The model under review builds one solid part; all positions refer to its coordinate system, in mm. A direction names the side the tool comes from. Round coordinates to 2 decimals unless told otherwise and drop trailing zeros. Order: outer loops, then holes, each group sorted by start corner. A loop starts at its lowest first (then second) coordinate and runs counter-clockwise, first axis right, second up.
1) Consider section D-D (y = 0). Give the number of separate pieces and of enclosed holes in the cut face, then the cut area to 3 significant figures.
2) Clearance check with flat-ended pins moving along their axes: P1, Ø1, axis at x = -20.5, y = 1, coming from the +Z side; P2, Ø1, axis at x = 3, y = -2, coming from the +Z side. State where each tip first meets the part, or that it passes through.
3) Consider section B-B (x = 9.5). Give the boundary of the cut face in (y, z).
4) Consider section C-C (z = 5.5). Give the boundary of the cut face in (x, y), then the cut area to 3 significant figures.
5) Consider section A-A (z = 18). Give the boundary of the cut face in (x, y).
6) To check wall thickness, follow L1, parallel to X at y = 0, z = 14.75; L2, parallel to Y at x = -18.5, z = 0.9; L3, parallel to Z at x = -21.5, y = 3.75. State the ranges of each line that lie inside material, in increasing order.
7) Machinability: for faces 4 (the face through (-5, 11, 12)), 5 (the face through (-16, 8.5, 8)), 6 (the face through (0, 0, 4)), 7 (the face through (10.63, -2.82, 15.67)), which of the approach directions +Z, -Z, +X, -X, +Y, -Y give a long, thin tool a straight path to every point of the face, cutting with its end or side? Answer none if there is none.
8) Mouldability with a two-part tool opening along X and no side actions: class faces 1 (the face through (20.4, 4.19, 9.98)), 2 (the face through (0, 0, 0)), 3 (the face through (32.5, 0, 10)) as pulls with the +X half, pulls with the -X half, needs draft (parallel to the pull), parting line crosses it, or undercut.
from build123d import *

# Parameters (mm, degrees)
SKETCH_W             = 65
SKETCH_H             = 24.999
PAD_DEPTH            = 19.999
POCKET_DEPTH         = 20.9992
POCKET001_DEPTH      = 20.9992
SKETCH003_R          = 10.9995
POCKET002_DEPTH      = 15.9992
SKETCH004_W          = 9.9995
SKETCH004_H          = 15.9992
POCKET003_DEPTH      = 12.5005
POCKET003_DEPTH_BACK = -12.5005
SKETCH005_R          = 3
POCKET004_DEPTH      = 20
CHAMFER_SIZE         = 1.5


with BuildPart() as part:
    # Sketch → Pad (new body)
    with BuildSketch(Plane.XY):
        Rectangle(SKETCH_W, SKETCH_H)
    extrude(amount=PAD_DEPTH)

    # Sketch001 → Pocket (cut)
    with BuildSketch(Plane.XZ.offset(-8.4997)):
        Polygon((0, 3.9998), (-30.5, 3.9998), (-30.5, 6.9996), (0, 15.9992), align=None)
    extrude(amount=POCKET_DEPTH, mode=Mode.SUBTRACT)

    # Sketch002 → Pocket001 (cut)
    with BuildSketch(Plane.XZ.offset(8.4997)):
        Polygon((0, 3.9998), (0, 15.9992), (30.5, 6.9996), (30.5, 3.9998), align=None)
    extrude(amount=-POCKET001_DEPTH, mode=Mode.SUBTRACT)

    # Sketch003 → Pocket002 (cut)
    with BuildSketch(Plane.XY.offset(19.999)):
        Circle(SKETCH003_R)
    extrude(amount=-POCKET002_DEPTH, mode=Mode.SUBTRACT)

    # Sketch004 → Pocket003 (cut, two sides)
    with BuildSketch(Plane.XZ) as pocket003_sk:
        with Locations((0, 11.9994)):
            Rectangle(SKETCH004_W, SKETCH004_H)
    extrude(amount=-POCKET003_DEPTH, mode=Mode.SUBTRACT)
    extrude(pocket003_sk.sketch, amount=-POCKET003_DEPTH_BACK, mode=Mode.SUBTRACT)

    # Sketch005 → Pocket004 (cut, through all)
    with BuildSketch(Plane.XY.offset(19.999)):
        with Locations((-18.5, 0)):
            Circle(SKETCH005_R)
        with Locations((18.5, 0)):
            Circle(SKETCH005_R)
    extrude(amount=-POCKET004_DEPTH, mode=Mode.SUBTRACT)

    # Chamfer
    chamfer_edges = [part.edges().sort_by_distance(p)[0] for p in [
        (-21.5, 0, 3.9998),
        (15.5, 0, 3.9998),
    ]]
    chamfer(chamfer_edges, length=CHAMFER_SIZE)


solid = part.part
Answer below:
1. separate pieces: 5
1. enclosed holes: 0
1. area: 553 mm2
2. P1: passes through
2. P2: stops at z = 4
3. outline: (-12.5, 0) - (12.5, 0) - (12.5, 4) - (-8.5, 4) - (-8.5, 13.2) - (-5.54, 13.2) - (-5.54, 20) - (-12.5, 20) - close; (5.54, 13.2) - (12.5, 13.2) - (12.5, 20) - (5.54, 20) - close
4. outline: (-32.5, -12.5) - (-30.5, -12.5) - (-30.5, 8.5) - (-6.98, 8.5) arc R11 cw to (-5, 9.8) - (-5, 12.5) - (-32.5, 12.5) - close; (5, -12.5) - (32.5, -12.5) - (32.5, 12.5) - (30.5, 12.5) - (30.5, -8.5) - (6.98, -8.5) arc R11 cw to (5, -9.8) - close
4. area: 301 mm2
5. outline: (-32.5, -12.5) - (-5, -12.5) - (-5, -9.8) arc R11 cw to (-5, 9.8) - (-5, 12.5) - (-32.5, 12.5) - close; (5, -12.5) - (32.5, -12.5) - (32.5, 12.5) - (5, 12.5) - (5, 9.8) arc R11 cw to (5, -9.8) - close; hole circle Ø6 at (-18.5, 0); hole circle Ø6 at (18.5, 0)
6. L1: x = -32.5 to -21.5, -15.5 to -11, 11 to 15.5, 21.5 to 32.5
6. L2: y = -12.5 to -3, 3 to 12.5
6. L3: z = 0 to 4, 9.66 to 20
7. face 4: +Z, +Y, -Y
7. face 5: -Y
7. face 6: none
7. face 7: +Z
8. face 1: undercut
8. face 2: needs draft
8. face 3: pulls with the +X half
